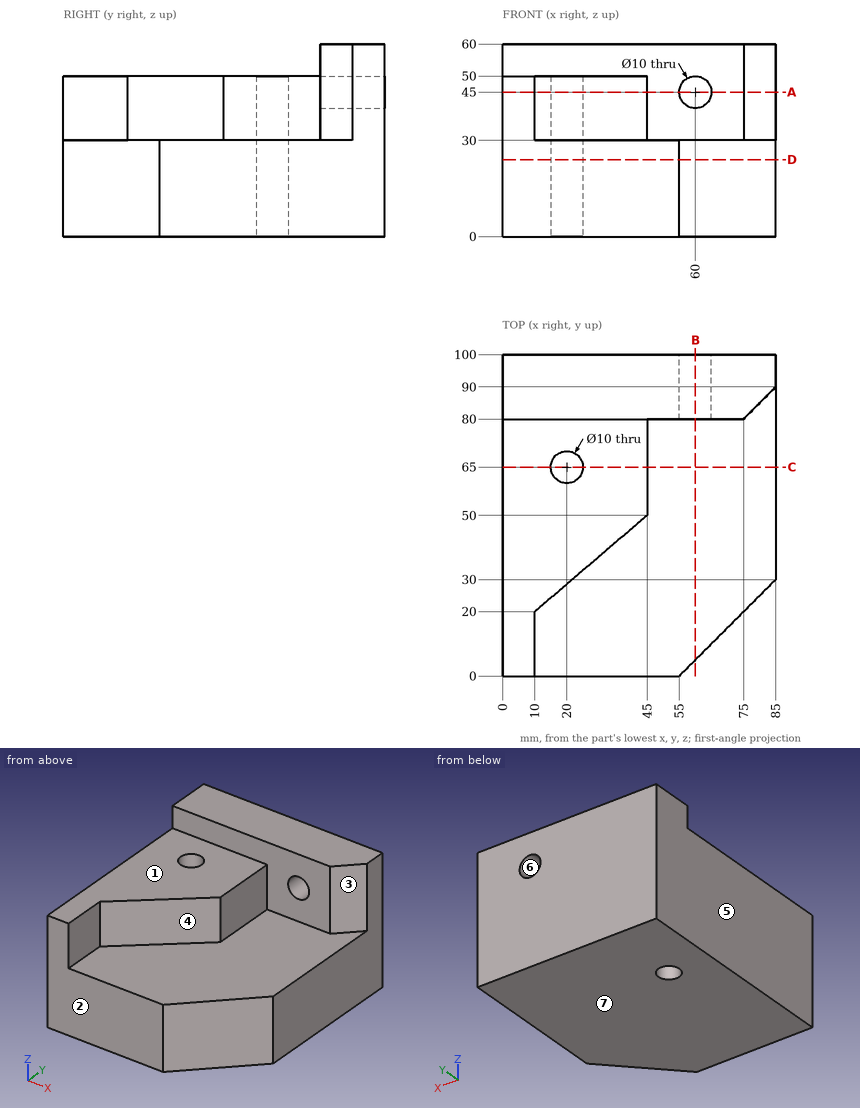
Here's the drawing with two shaded views (mm, measured from the low corner). I have some questions. A direction names the side the tool comes from. Coordinates: 2 decimals unless noted, no trailing zeros. Write each loop counter-clockwise with the first axis right and the second up, starting at its lowest first coordinate (ties: lowest second). Pieces come first, ordered by that corner, then holes. Notation, with made-up numbers: M -16,69.5 L 4,69.5 A20 cw 4,89.5 Z; hole C 33,5 d3. An arc over 180 degrees is marked long. Write item = value, one per line. Start each with the question number.
Q1. I'm going to push flat-ended pins straight in: pin 1 (10 mm diameter, centred on y = 60, z = 44, fed in from +X); pin 2 (22.5 mm diameter, centred on x = 28.5, y = 48.5, fed in from +Z); pin 3 (3 mm diameter, centred on x = 18.5, z = 47, fed in from -Y). Where does each tip first touch, or does it pass through?
Q2. If we section it at B-B, the plane x = 60: Write out the boundary of the cut face in (y, z).
Q3. If I drill on L1, parallel to Y at x = 20, z = 28; L2, parallel to X at y = 65, z = 18; L3, parallel to Z at x = 60, y = 86.5, over which ranges is the centre line in solid material (lowest first)? Write a range as [from, to].
Q4. On a 3-axis mill with a long thin cutter (end or side, diameter ignored), from which of +Z, -Z, +X, -X, +Y, -Y can I reach the whole of each face in a straight line? I mean the marked faces 1, 2 and 3. Say none if no direction works.
Q5. If we section it at C-C, the plane y = 65: Write out the boundary of the cut face in (x, z), then the cut area to 3 significant figures.
Q6. If we section it at A-A, the plane z = 45: Write out the boundary of the cut face in (x, y), then the cut area to 3 significant figures.
Q7. Thinking about a two-plate mould opening in X: for the marked faces 4, 5, 6 and 7, which applies, released by +X, released by -X, zero draft, split by the parting line, or undercut?
Q8. If we section it at D-D, the plane z = 24: Write out the boundary of the cut face in (x, y), then the cut area to 3 significant figures.
Check sheet entries:
q1.pin_1 = 45
q1.pin_2 = 50
q1.pin_3 = 26
q2.outline = M 5,0 L 100,0 L 100,40 L 80,40 L 80,30 L 5,30 Z; M 80,50 L 100,50 L 100,60 L 80,60 Z
q3.L1 = [0, 60], [70, 100]
q3.L2 = [0, 15], [25, 85]
q3.L3 = [0, 40], [50, 60]
q4.face_1 = +Z, +X, -X, -Y
q4.face_2 = +Z, -Z, +X, -X, -Y
q4.face_3 = +Z, +X, -Y
q5.outline = M 0,0 L 15,0 L 15,50 L 0,50 Z; M 25,0 L 85,0 L 85,30 L 45,30 L 45,50 L 25,50 Z
q5.area = 2,950 mm²
q6.outline = M 0,0 L 10,0 L 10,20 L 45,50 L 45,80 L 55,80 L 55,100 L 0,100 Z; M 65,80 L 75,80 L 85,90 L 85,100 L 65,100 Z; hole C 20,65 d10
q6.area = 3,750 mm²
q7.face_4 = released by +X
q7.face_5 = released by -X
q7.face_6 = undercut
q7.face_7 = zero draft
q8.outline = M 0,0 L 55,0 L 85,30 L 85,100 L 0,100 Z; hole C 20,65 d10
q8.area = 7,970 mm²
